Can you work these out from the drawing? Everything is in mm from the part's minimum corner. A direction names the side the tool comes from. Give positions to 0.01 mm unless a question says otherwise; leave off trailing zeros. Loops run counter-clockwise (first coordinate to the right, second up) from the corner with the lowest first, then second, coordinate; pieces in that order, holes last. Notation, with made-up numbers: (-1, 73) -> (27, 73) arc R20 ccw to (27, 85) -> close; hole circle Ø2 at (56, 16.5). An arc over 180 degrees is marked (long way). Return JSON: item names as keys, results as strings. Group by question number.
Q1. Suppose I cut it at A-A, the plane x = 36.5. Please give me the cut outline in (y, z).
Q2. Which directions (+Z, -Z, +X, -X, +Y, -Y) give clear straight access to the entire face, cutting with the end or side of a thin tool? Please do the marked faces 4 and 5.
Q3. I need wall thicknesses on line 1 along Y through (x, z) = (36.5, 4); line 2 along Z through (x, y) = (32, 67.5); line 3 along Y through (x, z) = (27.5, 1.5). Which ranges of each line are inside material? Lowest first, please. Write a range as [from, to].
Q4. Thinking about a two-plate mould opening in X: for the marked faces 1, 2 and 3, which applies, pulls with the +X half, pulls with the -X half, needs draft (parallel to the pull), parting line crosses it, or undercut?
Q5. Will these pins go through, and if not, where does the flat tip stop? pin 1 (1.6 mm diameter, centred on x = 16.5, z = 6, fed in from -Y) (3 decimals); pin 2 (4 mm diameter, centred on x = 38, y = 30, fed in from -Z); pin 3 (1.8 mm diameter, centred on y = 36, z = 7.5, fed in from -X); pin 4 (2 mm diameter, centred on x = 22.5, z = 4.5, fed in from +Y).
Q6. Suppose I cut it at B-B, the plane y = 36.5. Please give me the cut outline in (x, z).
Q7. Suppose I cut it at C-C, the plane z = 1.5. Please give me the cut outline in (x, y).
Q8. Suppose I cut it at D-D, the plane y = 44.5. Please give me the cut outline in (x, z), and give its area (3 significant figures).
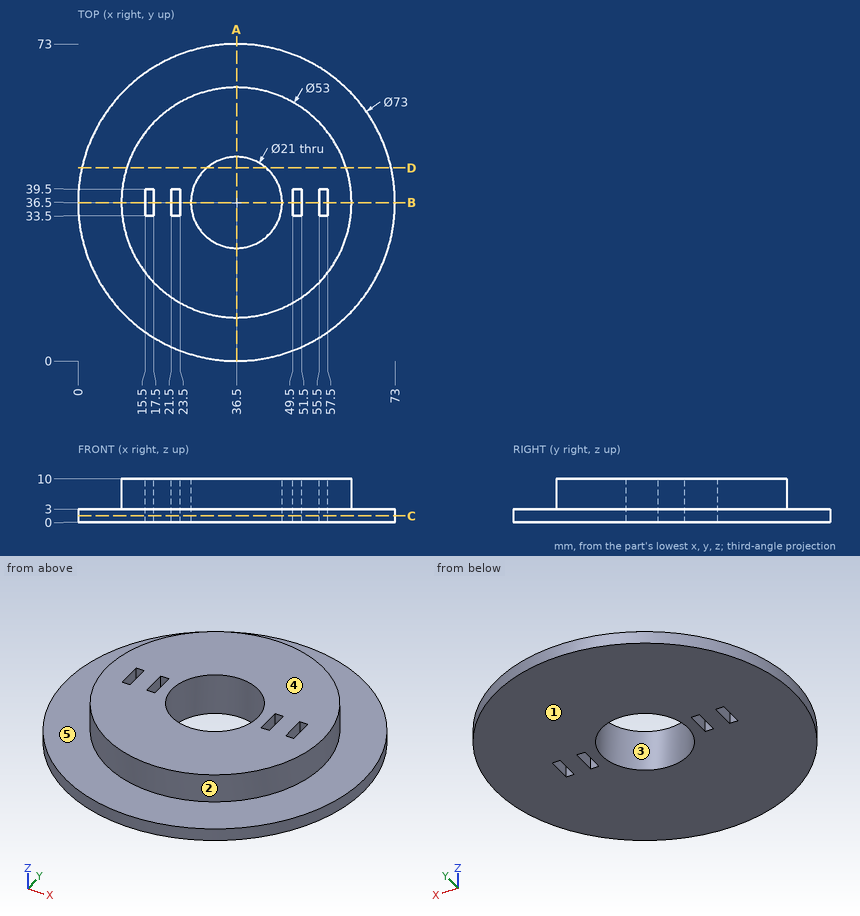
Ans:
{
 "1": {"outline": "(0, 0) -> (26, 0) -> (26, 10) -> (10, 10) -> (10, 3) -> (0, 3) -> close; (47, 0) -> (73, 0) -> (73, 3) -> (63, 3) -> (63, 10) -> (47, 10) -> close"},
 "2": {"face 4": "+Z, +X, -X, +Y, -Y", "face 5": "+Z"},
 "3": {"line 1": "y = [10, 26], [47, 63]", "line 2": "z = [0, 3]", "line 3": "y = [1.13, 31.09], [41.91, 71.87]"},
 "4": {"face 1": "needs draft", "face 2": "parting line crosses it", "face 3": "undercut"},
 "5": {"pin 1": "stops at y = 18.235", "pin 2": "passes through", "pin 3": "stops at x = 10", "pin 4": "stops at y = 59.59"},
 "6": {"outline": "(0, 0) -> (15.5, 0) -> (15.5, 10) -> (10, 10) -> (10, 3) -> (0, 3) -> close; (17.5, 0) -> (21.5, 0) -> (21.5, 10) -> (17.5, 10) -> close; (23.5, 0) -> (26, 0) -> (26, 10) -> (23.5, 10) -> close; (47, 0) -> (49.5, 0) -> (49.5, 10) -> (47, 10) -> close; (51.5, 0) -> (55.5, 0) -> (55.5, 10) -> (51.5, 10) -> close; (57.5, 0) -> (73, 0) -> (73, 3) -> (63, 3) -> (63, 10) -> (57.5, 10) -> close"},
 "7": {"outline": "circle Ø73 at (36.5, 36.5); hole (15.5, 33.5) -> (17.5, 33.5) -> (17.5, 39.5) -> (15.5, 39.5) -> close; hole (21.5, 33.5) -> (23.5, 33.5) -> (23.5, 39.5) -> (21.5, 39.5) -> close; hole circle Ø21 at (36.5, 36.5); hole (49.5, 33.5) -> (51.5, 33.5) -> (51.5, 39.5) -> (49.5, 39.5) -> close; hole (55.5, 33.5) -> (57.5, 33.5) -> (57.5, 39.5) -> (55.5, 39.5) -> close"},
 "8": {"outline": "(0.89, 0) -> (29.7, 0) -> (29.7, 10) -> (11.24, 10) -> (11.24, 3) -> (0.89, 3) -> close; (43.3, 0) -> (72.11, 0) -> (72.11, 3) -> (61.76, 3) -> (61.76, 10) -> (43.3, 10) -> close", "area": "431 mm^2"}
}
